Part model, mm, in its own coordinate system. Round coordinates to 2 decimals unless told otherwise and drop trailing zeros. Write each loop counter-clockwise with the first axis right and the second up, starting at its lowest first coordinate (ties: lowest second). Pieces come first, ordered by that corner, then holes. Notation, with made-up numbers: M 77.5,29 L 115.5,29 A20 cw 115.5,51 Z; hole C 47,-21.75 d6. An arc over 180 degrees is marked long. Use a Markdown table: item, result. Add a question column.
1) Slice it at D-D on y = -1. Write the cut outline in (x, z).
2) Slice it at A-A on z = 1.15. Write the cut outline in (x, y).
3) Wall check: probe 1 along X at (y, z) = (-10.75, 1.65); probe 2 along X at (y, z) = (-9.5, 0.9); probe 3 along Y at (x, z) = (69, 1.15). Give the ranges that are in metal, low to high.
4) Slice it at C-C on x = 2.5. Write the cut outline in (y, z).
5) Drop a flat-ended pin along its axis: P1, Ø2, axis at x = 47, y = -7.5, coming from the -Z side. Give the stop position or say it passes through.
6) Slice it at B-B on y = -6.75. Write the cut outline in (x, z) (3 decimals).
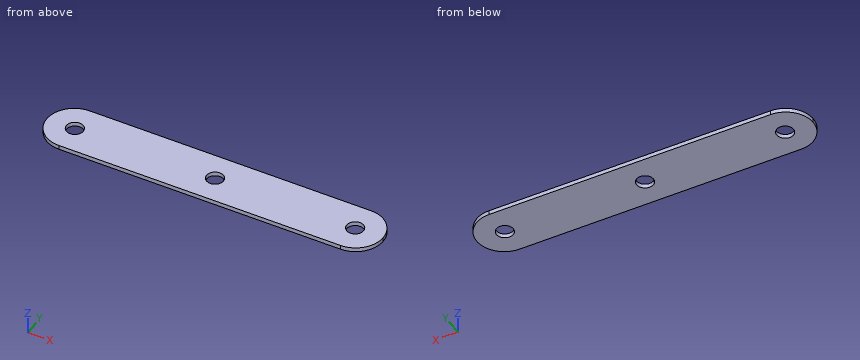
```python
from build123d import *

# Parameters (mm, degrees)
F0_R     = 4
F1_DEPTH = 2


with BuildPart() as f1:
    # F0 (on Top) → F1 (new body)
    with BuildSketch(Plane.XY):
        with BuildLine():
            Line((72.098875, 4.53313), (-61.901125, 4.53313))
            ThreePointArc((-61.901125, 4.53313), (-71.093513, 0.725518), (-74.901125, -8.46687))
            ThreePointArc((-74.901125, -8.46687), (-71.093513, -17.659259), (-61.901125, -21.46687))
            Line((-61.901125, -21.46687), (72.098875, -21.46687))
            ThreePointArc((72.098875, -21.46687), (81.291263, -17.659259), (85.098875, -8.46687))
            ThreePointArc((85.098875, -8.46687), (81.291263, 0.725518), (72.098875, 4.53313))
        make_face()
        with Locations((-61.628222, -8.46687)):
            Circle(F0_R, mode=Mode.SUBTRACT)
        with Locations((5.098875, -8.46687)):
            Circle(F0_R, mode=Mode.SUBTRACT)
        with Locations((71.825972, -8.46687)):
            Circle(F0_R, mode=Mode.SUBTRACT)
    extrude(amount=F1_DEPTH)


solid = f1.part
```
Entries:
| question | item | result |
|---|---|---|
| 1 | outline | M -72.54,0 L 82.74,0 L 82.74,2 L -72.54,2 Z |
| 2 | outline | M -74.9,-8.47 A13 ccw -61.9,-21.47 L 72.1,-21.47 A13 ccw 85.1,-8.47 A13 ccw 72.1,4.53 L -61.9,4.53 A13 ccw Z; hole C -61.63,-8.47 d8; hole C 5.1,-8.47 d8; hole C 71.83,-8.47 d8 |
| 3 | probe 1 | x = -74.7 to -64.91, -58.34 to 1.81, 8.38 to 68.54, 75.11 to 84.9 |
| 3 | probe 2 | x = -74.86 to -65.49, -57.76 to 1.23, 8.96 to 67.96, 75.69 to 85.06 |
| 3 | probe 3 | y = -21.47 to -11.3, -5.64 to 4.53 |
| 4 | outline | M -21.47,0 L -11.51,0 L -11.51,2 L -21.47,2 Z; M -5.43,0 L 4.53,0 L 4.53,2 L -5.43,2 Z |
| 5 | P1 | stops at z = 0 |
| 6 | outline | M -74.787,0 L -65.241,0 L -65.241,2 L -74.787,2 Z; M -58.015,0 L 1.486,0 L 1.486,2 L -58.015,2 Z; M 8.712,0 L 68.213,0 L 68.213,2 L 8.712,2 Z; M 75.439,0 L 84.985,0 L 84.985,2 L 75.439,2 Z |
